```python
from build123d import *

# Parameters (mm, degrees)
SKETCH1_R              = 100
SKETCH1_R_2            = 98
BOSS_EXTRUDE1_DEPTH    = 80
CUT_EXTRUDE1_START     = -100.0000001
CUT_EXTRUDE1_OUTLINE_R = 1.65
CUT_EXTRUDE1_DEPTH     = 200.000000187
CIRPATTERN1_COUNT      = 3


# Read off the part's stored shape, not the designer's step: Cut-Extrude1
with BuildPart() as part:
    # Sketch1 → Boss-Extrude1 (new body)
    with BuildSketch(Plane(origin=(0, 0, 0), x_dir=(1, 0, 0), z_dir=(0, 1, 0))):
        with Locations(Location((0, 0, 0), (0, 0, 270))):
            Circle(SKETCH1_R)
        with Locations(Location((0, 0, 0), (0, 0, 270))):
            Circle(SKETCH1_R_2, mode=Mode.SUBTRACT)
    extrude(amount=BOSS_EXTRUDE1_DEPTH)

    # Cut-Extrude1 outline → Cut-Extrude1 (cut)
    with BuildSketch(Plane.XY.offset(CUT_EXTRUDE1_START)):
        with Locations((0, 70)):
            Circle(CUT_EXTRUDE1_OUTLINE_R)
    cut_extrude1 = extrude(amount=CUT_EXTRUDE1_DEPTH, mode=Mode.SUBTRACT)

    # CirPattern1: Cut-Extrude1 ×3 about axis
    cirpattern1_axis = Axis((0, 80, 0), (0, -1, 0))
    for i in range(1, CIRPATTERN1_COUNT):
        add(cut_extrude1.rotate(cirpattern1_axis, i * 360 / CIRPATTERN1_COUNT), mode=Mode.SUBTRACT)


solid = part.part
```
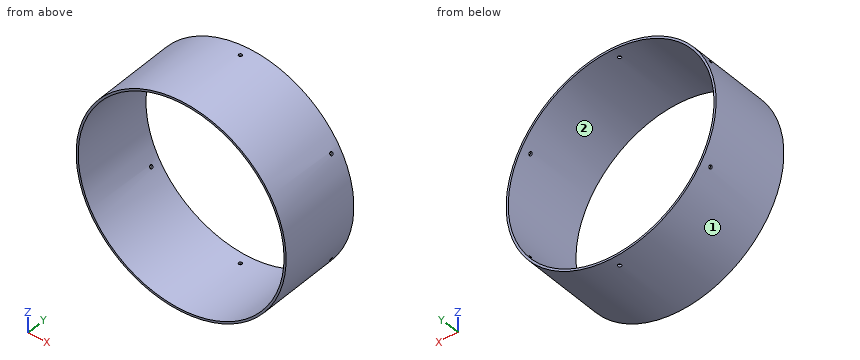
Here's how the part is built. I have some questions about the finished solid (model axes, mm). Face numbers are marked on the shaded views. Coordinates: 2 decimals unless noted, no trailing zeros. Order: outer loops, then holes, each group sorted by start corner. A loop starts at its lowest first (then second) coordinate and runs counter-clockwise, first axis right, second up. Notation, with made-up numbers: (15.25, -37) -> (25.25, -37) arc R22 ccw to (25.25, -7) -> close; hole circle Ø4 at (-20, 65). An arc over 180 degrees is marked (long way). Return JSON: item names as keys, results as strings.
1) If we section it at A-A on z = 0: List the corners of the cut face in (x, y) for me.
Conclusion:
{"outline": "(-100, 0) -> (-98, 0) -> (-98, 80) -> (-100, 80) -> close; (98, 0) -> (100, 0) -> (100, 80) -> (98, 80) -> close"}
2) If we section it at C-C on y = 62: List the corners of the cut face in (x, z) for me.
Conclusion:
{"outline": "circle Ø200 at (0, 0); hole circle Ø196 at (0, 0)"}
3) If we section it at B-B on x = 4.5: List the corners of the cut face in (y, z) for me.
Conclusion:
{"outline": "(0, -99.9) -> (80, -99.9) -> (80, -97.9) -> (0, -97.9) -> close; (0, 97.9) -> (80, 97.9) -> (80, 99.9) -> (0, 99.9) -> close"}
4) If I drill on probe 1 along X at (y, z) = (24, 0); probe 2 along Y at (x, z) = (0, 99), over which ranges is the centre line in solid material (lowest first)?
Conclusion:
{"probe 1": "x = -100 to -98, 98 to 100", "probe 2": "y = 0 to 68.35, 71.65 to 80"}
5) I'm going to push flat-ended pins straight in: P1, Ø4, axis at y = 36, z = 6.5, coming from the -X side; P2, Ø3, axis at x = 0, y = 70, coming from the -Z side; P3, Ø4, axis at y = 43.5, z = 50.5, coming from the -X side; P4, Ø1, axis at y = 31.5, z = -59, coming from the +X side. Where does each tip first touch, or does it pass through?
Conclusion:
{"P1": "stops at x = -99.9", "P2": "passes through", "P3": "stops at x = -87.45", "P4": "stops at x = 81.1"}
6) Thinking about a two-plate mould opening in Z: for the marked faces 1 and 2, which applies, +Z half, -Z half, draft (parallel to the pull), parting line (faces both ways), or undercut?
Conclusion:
{"face 1": "parting line", "face 2": "undercut"}
